Check sheet for the drawn part. Datum: minimum x, y, z corner. Units: mm. A direction names the side the tool comes from. Give positions to 0.01 mm unless a question says otherwise; leave off trailing zeros. Write each loop counter-clockwise with the first axis right and the second up, starting at its lowest first coordinate (ties: lowest second). Pieces come first, ordered by that corner, then holes. Notation, with made-up numbers: (4.25, 68.25) -> (61.25, 68.25) arc R31 ccw to (61.25, 93.25) -> close; hole circle Ø9 at (14.5, -29). An arc over 180 degrees is marked (long way). Answer as CSV lines item,"result". Start each with the question number.
1) Sectioned sample at C-C on z = 38. Record the cut outline in (x, y).
2) Material ranges on L1, parallel to Y at x = 6.25, z = 44 (1 decimal); L2, parallel to Z at x = 5, y = 8; L3, parallel to Z at x = 5, y = 6.5, recorded low to high.
3) Gauge pin test, flat ends, axial feed: pin 1 Ø3 at (x, y) = (8, 8.5) entering from +Z; pin 2 Ø2 at (y, z) = (7, 15) entering from -X; pin 3 Ø2 at (y, z) = (3, 28.5) entering from +X. Record the tip position at first contact, or that the pin passes through.
4) Sectioned sample at D-D on x = 5. Record the cut outline in (y, z) (3 decimals).
5) Sectioned sample at B-B on y = 1. Record the cut outline in (x, z), and give its area (3 significant figures).
6) Sectioned sample at A-A on x = 3.25. Record the cut outline in (y, z).
7) Tool access check on the marked faces 1 and 2. Record the directions out of +Z, -Z, +X, -X, +Y, -Y that give a thin tool (end or side, any length) a straight path to the whole face; none if there is none.
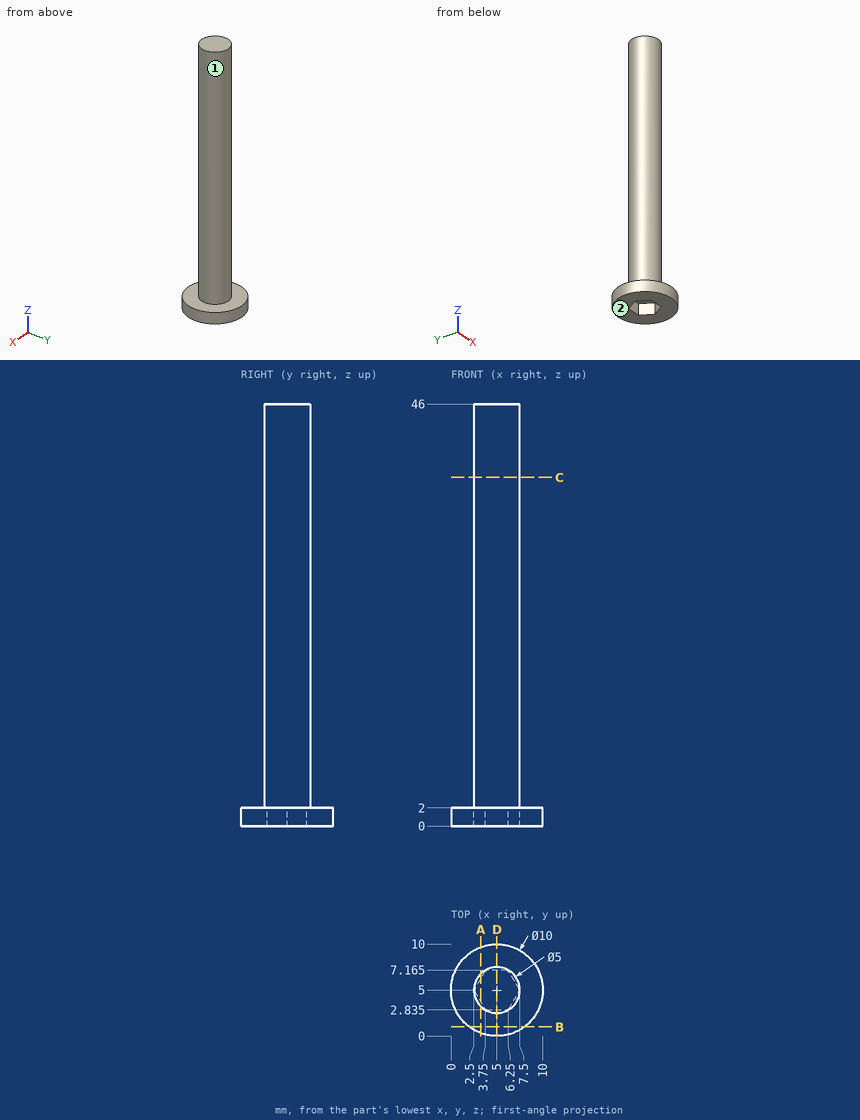
Ans:
1,outline,"circle Ø5 at (5, 5)"
2,L1,"y = 2.8 to 7.2"
2,L2,"z = 0 to 2"
2,L3,"z = 2 to 46"
3,pin 1,"stops at z = 2"
3,pin 2,"stops at x = 2.71"
3,pin 3,"stops at x = 7.29"
4,outline,"(0, 0) -> (2.835, 0) -> (2.835, 2) -> (7.165, 2) -> (7.165, 0) -> (10, 0) -> (10, 2) -> (7.5, 2) -> (7.5, 46) -> (2.5, 46) -> (2.5, 2) -> (0, 2) -> close"
5,outline,"(2, 0) -> (8, 0) -> (8, 2) -> (2, 2) -> close"
5,area,"12.0 mm²"
6,outline,"(0.32, 0) -> (3.7, 0) -> (3.7, 2) -> (6.3, 2) -> (6.3, 0) -> (9.68, 0) -> (9.68, 2) -> (6.79, 2) -> (6.79, 46) -> (3.21, 46) -> (3.21, 2) -> (0.32, 2) -> close"
7,face 1,"+Z"
7,face 2,"-Z, +X, -X, +Y, -Y"
